from build123d import *

# Parameters (mm, degrees)
F0_R      = 54.25
F0_R_2    = 25.4
F1_DEPTH  = 55
F3_START  = -20
F2_R      = 54.25
F2_R_2    = 46.35
F3_DEPTH  = 6.7
F4_R      = 54.25
F4_R_2    = 50.7
F5_DEPTH  = 48.5
F6_R      = 50.7
F6_R_2    = 43.4
F7_DEPTH  = 13.7
F8_R      = 1
F9_R      = 45
F9_R_2    = 25.4
F10_DEPTH = 6
F11_R     = 1


with BuildPart() as f1:
    # F0 (on Front) → F1 (new body)
    with BuildSketch(Plane.XZ):
        Circle(F0_R)
        Circle(F0_R_2, mode=Mode.SUBTRACT)
    extrude(amount=F1_DEPTH)

    # F2 (on face) → F3 (cut)
    with BuildSketch(Plane.XZ.offset(55).offset(F3_START)):
        Circle(F2_R)
        Circle(F2_R_2, mode=Mode.SUBTRACT)
    extrude(amount=-F3_DEPTH, mode=Mode.SUBTRACT)

    # F4 (on face) → F5 (cut)
    with BuildSketch(Plane.XZ.offset(55)):
        Circle(F4_R)
        Circle(F4_R_2, mode=Mode.SUBTRACT)
    extrude(amount=-F5_DEPTH, mode=Mode.SUBTRACT)

    # F6 (on face) → F7 (cut)
    with BuildSketch(Plane.XZ.offset(55)):
        Circle(F6_R)
        Circle(F6_R_2, mode=Mode.SUBTRACT)
    extrude(amount=-F7_DEPTH, mode=Mode.SUBTRACT)

    # F8
    f8_edges = [f1.edges().sort_by_distance(p)[0] for p in [
        (-25.4, -55, 0),
    ]]
    fillet(f8_edges, radius=F8_R)

    # F9 (on Front) → F10 (join)
    with BuildSketch(Plane.XZ):
        Circle(F9_R)
        Circle(F9_R_2, mode=Mode.SUBTRACT)
    extrude(amount=-F10_DEPTH)

    # F11
    f11_edges = [f1.edges().sort_by_distance(p)[0] for p in [
        (-45, 6, 0),
    ]]
    fillet(f11_edges, radius=F11_R)


solid = f1.part
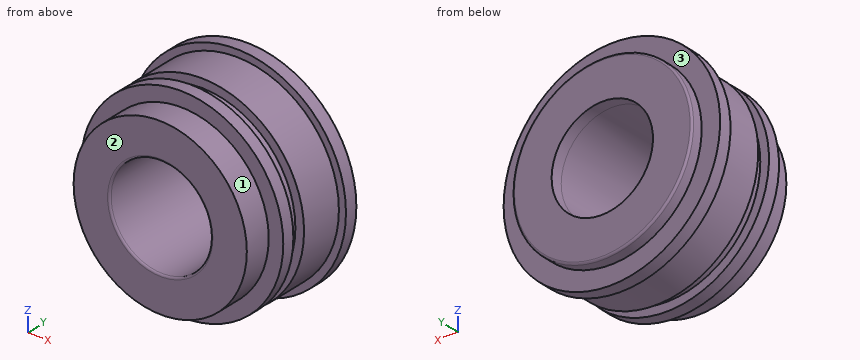
Can you work these out from the model? Positions are in its coordinate system, mm. Face numbers are marked on the shaded views. A direction names the side the tool comes from. Give positions to 0.01 mm unless a question says otherwise; leave off trailing zeros. Loops run counter-clockwise (first coordinate to the right, second up) from the corner with the lowest first, then second, coordinate; pieces in that order, holes last. Notation, with made-up numbers: M 18.25,78.25 L 74.25,78.25 A18 ccw 74.25,83.25 Z; hole C 1.25,45 d3. An arc over 180 degrees is marked long. One line per item, written item: value.
1) Please list where these lines run through material, in increasing order: line 1 (Z direction, x = 0, y = 1); line 2 (Z direction, x = 0, y = -17); line 3 (Y direction, x = -20, z = -50).
Geometry check:
line 1: z = -45 to -25.4, 25.4 to 45
line 2: z = -50.7 to -25.4, 25.4 to 50.7
line 3: y = -6.5 to 0
2) On a 3-axis mill with a long thin cutter (end or side, diameter ignored), from which of +Z, -Z, +X, -X, +Y, -Y can I reach the whole of each face in a straight line? I mean the marked faces 1, 2 and 3. Say none if no direction works.
Geometry check:
face 1: -Y
face 2: +Z, -Z, +X, -X, -Y
face 3: +Y
3) I'm going to push flat-ended pins straight in: pin 1 (6 mm diameter, centred on x = -31.5, y = -47.5, fed in from +Z); pin 2 (5 mm diameter, centred on x = -19.5, y = -2, fed in from +Z); pin 3 (2 mm diameter, centred on y = -0.5, z = 32.5, fed in from +X). Where does each tip first touch, or does it pass through?
Geometry check:
pin 1: stops at z = 32.73
pin 2: stops at z = 51.52
pin 3: stops at x = 44.17
4) Imagine slicing it at D-D on y = -45.5. Write out the boundary of the cut face in (x, z).
Geometry check:
outline: C 0,0 d86.8; hole C 0,0 d50.8
5) Imagine slicing it at C-C on y = -17. Write out the boundary of the cut face in (x, z), and give its area (3 significant figures).
Geometry check:
outline: C 0,0 d101.4; hole C 0,0 d50.8
area: 6,050 mm²
